```python
from build123d import *

# Parameters (mm, degrees)
BOSS_EXTRUDE1_DEPTH  = 370
CUT_EXTRUDE1_DEPTH   = 377.385766877
M5_CLEARANCE_HOLE1_D = 5.5
M8_CLEARANCE_HOLE1_D = 9
FILLET1_R            = 2
FILLET2_R            = 3.5
CUT_EXTRUDE2_DEPTH   = 373.141046534


with BuildPart() as part:
    # Sketch1 → Boss-Extrude1 (new body)
    with BuildSketch(Plane.XY):
        Polygon((0, 3.96875), (0, 0), (32.54375, 0), (32.54375, 23.01875), (28.575, 23.01875), (28.575, 3.96875), align=None)
        Polygon((-28.575, 23.01875), (-32.54375, 23.01875), (-32.54375, 0), (0, 0), (0, 3.96875), (-28.575, 3.96875), align=None)
    extrude(amount=BOSS_EXTRUDE1_DEPTH)

    # Sketch2 → Cut-Extrude1 (cut, through all)
    with BuildSketch(Plane.ZY.offset(32.54375)):
        Polygon((0, 3.96875), (32.995567884, 23.01875), (0, 23.01875), align=None)
        Polygon((370, 23.01875), (370, 3.96875), (337.004432116, 23.01875), align=None)
    extrude(amount=-CUT_EXTRUDE1_DEPTH, mode=Mode.SUBTRACT)

    # M5 Clearance Hole1 (through all)
    with Locations(Plane(origin=(0, 3.96875, 0), x_dir=(1, 0, 0), z_dir=(0, 1, 0))):
        with Locations((20, -360), (20, -320), (-20, -320), (-20, -360)):
            Hole(M5_CLEARANCE_HOLE1_D / 2)

    # M8 Clearance Hole1 (through all)
    with Locations(Plane(origin=(0, 3.96875, 0), x_dir=(1, 0, 0), z_dir=(0, 1, 0))):
        with Locations((0, -28)):
            Hole(M8_CLEARANCE_HOLE1_D / 2)

    # Fillet1
    fillet1_edges = [part.edges().sort_by_distance(p)[0] for p in [
        (28.575, 3.96875, 185),
        (-28.575, 3.96875, 185),
    ]]
    fillet(fillet1_edges, radius=FILLET1_R)

    # Fillet2
    fillet2_edges = [part.edges().sort_by_distance(p)[0] for p in [
        (32.54375, 0, 185),
        (-32.54375, 0, 185),
    ]]
    fillet(fillet2_edges, radius=FILLET2_R)

    # Sketch8 → Cut-Extrude2 (cut, through all)
    with BuildSketch(Plane.XZ):
        with BuildLine():
            Line((-32.54375, 366.5), (-32.54375, 370))
            Line((-32.54375, 370), (-29.04375, 370))
            ThreePointArc((-29.04375, 370), (-31.518623734, 368.974873734), (-32.54375, 366.5))
        make_face()
        with BuildLine():
            Line((29.04375, 370), (32.54375, 370))
            Line((32.54375, 370), (32.54375, 366.5))
            ThreePointArc((32.54375, 366.5), (31.518623734, 368.974873734), (29.04375, 370))
        make_face()
    extrude(amount=-CUT_EXTRUDE2_DEPTH, mode=Mode.SUBTRACT)


solid = part.part
```
Work out the finished part from the listing and answer in its coordinate system (mm). A direction names the side the tool comes from. Round coordinates to 2 decimals unless told otherwise and drop trailing zeros. Loops run counter-clockwise (first coordinate to the right, second up) from the corner with the lowest first, then second, coordinate; pieces in that order, holes last.
(1) The part is cut by section C-C, the plane y = 19. Give the vertices of the cut face in (x, z) (3 decimals).
Computed values:
outline: (-32.544, 26.035) - (-28.575, 26.035) - (-28.575, 343.965) - (-32.544, 343.965) - close; (28.575, 26.035) - (32.544, 26.035) - (32.544, 343.965) - (28.575, 343.965) - close
(2) The part is cut by section B-B, the plane z = 28. Give the vertices of the cut face in (x, y) (3 decimals).
Computed values:
outline: (-32.544, 3.5) arc R3.5 ccw to (-29.044, 0) - (-4.5, 0) - (-4.5, 3.969) - (-26.575, 3.969) arc R2 cw to (-28.575, 5.969) - (-28.575, 20.135) - (-32.544, 20.135) - close; (4.5, 0) - (29.044, 0) arc R3.5 ccw to (32.544, 3.5) - (32.544, 20.135) - (28.575, 20.135) - (28.575, 5.969) arc R2 cw to (26.575, 3.969) - (4.5, 3.969) - close
(3) The part is cut by section D-D, the plane z = 271.5. Give the vertices of the cut face in (x, y) (3 decimals).
Computed values:
outline: (-32.544, 3.5) arc R3.5 ccw to (-29.044, 0) - (29.044, 0) arc R3.5 ccw to (32.544, 3.5) - (32.544, 23.019) - (28.575, 23.019) - (28.575, 5.969) arc R2 cw to (26.575, 3.969) - (-26.575, 3.969) arc R2 cw to (-28.575, 5.969) - (-28.575, 23.019) - (-32.544, 23.019) - close
(4) Find the intervals of material crossed by L1, parallel to Z at x = -20, y = 2.65; L2, parallel to X at y = 3.1, z = 320; L3, parallel to X at y = 5.5, z = 162.5, in increasing order.
Computed values:
L1: z = 0 to 317.25, 322.75 to 357.25, 362.75 to 370
L2: x = -32.52 to -22.75, -17.25 to 17.25, 22.75 to 32.52
L3: x = -32.54 to -28.52, 28.52 to 32.54
(5) The part is cut by section A-A, the plane x = 0. Give the vertices of the cut face in (y, z).
Computed values:
outline: (0, 0) - (3.97, 0) - (3.97, 23.5) - (0, 23.5) - close; (0, 32.5) - (3.97, 32.5) - (3.97, 370) - (0, 370) - close
(6) For faces 4 (the flat face through (0, 3.969, 182)), 5 (the flat face through (0, 0, 182)), determine the directions among +Z, -Z, +X, -X, +Y, -Y from which every point of the face is accessible in a straight line to the end or side of a thin tool.
Computed values:
face 4: +Z, -Z, +Y
face 5: +Z, -Z, +X, -X, -Y
(7) This flat-tipped pin is pushed along its axis until it touches: P1, Ø1, axis at x = -21.5, z = 154, coming from the +Y side. Where does it stop, or does it pass through?
Computed values:
P1: stops at y = 3.97
(8) The mould has two halves that part along X. Classify faces 1 (the flat face through (-30.26, 13.36, 353.73)), 2 (the flat face through (32.544, 13, 181)), 3 (the cylindrical face through (0.98, 1.96, 32.39)): pulls with the +X half, pulls with the -X half, needs draft (parallel to the pull), parting line crosses it, or undercut.
Computed values:
face 1: needs draft
face 2: pulls with the +X half
face 3: undercut
